Build history of the part. All positions in model axes, mm. A direction names the side the tool comes from. Give positions to 0.01 mm unless a question says otherwise; leave off trailing zeros. Order: outer loops, then holes, each group sorted by start corner. A loop starts at its lowest first (then second) coordinate and runs counter-clockwise, first axis right, second up. Notation, with made-up numbers: (-32, -33.75) -> (-16, -33.75) arc R13 cw to (-16, -29.75) -> close; hole circle Ø10 at (53.25, 40.5). An arc over 180 degrees is marked (long way). One line per item, written item: value. Start each with the question number.
(1) Saw through at A-A on x = 0. Give the cut face in (y, z) (1 decimal).
(2) Two-plate mould, pull along Z, no slides. Class faces 3 (the flat face through (8, 1.905, 208)), 4 (the flat face through (-3, 4.064, -3)): +Z half, -Z half, draft (parallel to the pull), parting line (faces both ways), or undercut.
(3) Pin check, flat tips, straight feed: pin 1 (2.5 mm diameter, centred on x = -23.57, z = 222.46, fed in from +Y); pin 2 (6.5 mm diameter, centred on x = -15, z = 167.17, fed in from -Y). Stop position of each tip, or through.
(4) Which spindle directions (+Z, -Z, +X, -X, +Y, -Y) get a long thin tool onto all of the face, cutting with end or side? Do faces 1 (the cylindrical face through (-193.461, 2.969, -209.304)), 2 (the cylindrical face through (184.75, 0.94, -185.92)). Say none if no direction does.
(5) Probe line 1 (X direction, y = 2.55, z = -199); line 2 (X direction, y = 2.25, z = -104); line 3 (Z direction, x = 24.5, y = 1.4). List the from-to ranges inside material, lowest first.
```python
from build123d import *

# Parameters (mm, degrees)
SKETCH1_W                                           = 457.2
SKETCH1_H                                           = 457.2
BOSS_EXTRUDE1_DEPTH                                 = 4.064
SKETCH2_R                                           = 19.177
CUT_EXTRUDE1_DEPTH                                  = 1.905
CUT_EXTRUDE2_REACH                                  = 4.159
SKETCH3_R                                           = 11.7475
F_10_32_TAPPED_HOLE1_D                              = 4.0386
F_10_32_TAPPED_HOLE2_D                              = 4.0386
CBORE_FOR_10_BINDING_HEAD_MACHINE_SCREW_D           = 5.1054
CBORE_FOR_10_BINDING_HEAD_MACHINE_SCREW_CBORE_D     = 11.1125
CBORE_FOR_10_BINDING_HEAD_MACHINE_SCREW_CBORE_DEPTH = 3.1242
F_1_4_0_25_DIAMETER_HOLE1_D                         = 6.35


with BuildPart() as part:
    # Sketch1 → Boss-Extrude1 (new body)
    with BuildSketch(Plane(origin=(0, 0, 0), x_dir=(1, 0, 0), z_dir=(0, 1, 0))):
        Rectangle(SKETCH1_W, SKETCH1_H)
    extrude(amount=BOSS_EXTRUDE1_DEPTH)

    # Sketch2 → Cut-Extrude1 (cut)
    with BuildSketch(Plane.XZ):
        with Locations((0, 198.882)):
            Circle(SKETCH2_R)
        with Locations((-198.882, -198.882)):
            Circle(SKETCH2_R)
        with Locations((198.882, -198.882)):
            Circle(SKETCH2_R)
    extrude(amount=-CUT_EXTRUDE1_DEPTH, mode=Mode.SUBTRACT)

    # Sketch3 → Cut-Extrude2 (cut, up to next)
    with BuildSketch(Plane.XZ.offset(-1.905), mode=Mode.PRIVATE) as cut_extrude2_sk1:
        with Locations((0, 198.882)):
            Circle(SKETCH3_R)
    cut_extrude2_tool1 = extrude(cut_extrude2_sk1.sketch, amount=-CUT_EXTRUDE2_REACH, mode=Mode.PRIVATE) & part.part
    add(cut_extrude2_tool1.solids().sort_by_distance((0, 1.905, 198.882))[0], mode=Mode.SUBTRACT)
    # Sketch3 → Cut-Extrude2 (cut, up to next)
    with BuildSketch(Plane.XZ.offset(-1.905), mode=Mode.PRIVATE) as cut_extrude2_sk2:
        with Locations((-198.882, -198.882)):
            Circle(SKETCH3_R)
    cut_extrude2_tool2 = extrude(cut_extrude2_sk2.sketch, amount=-CUT_EXTRUDE2_REACH, mode=Mode.PRIVATE) & part.part
    add(cut_extrude2_tool2.solids().sort_by_distance((-198.882, 1.905, -198.882))[0], mode=Mode.SUBTRACT)
    # Sketch3 → Cut-Extrude2 (cut, up to next)
    with BuildSketch(Plane.XZ.offset(-1.905), mode=Mode.PRIVATE) as cut_extrude2_sk3:
        with Locations((198.882, -198.882)):
            Circle(SKETCH3_R)
    cut_extrude2_tool3 = extrude(cut_extrude2_sk3.sketch, amount=-CUT_EXTRUDE2_REACH, mode=Mode.PRIVATE) & part.part
    add(cut_extrude2_tool3.solids().sort_by_distance((198.882, 1.905, -198.882))[0], mode=Mode.SUBTRACT)

    # #10-32 Tapped Hole1 (through all)
    with Locations(Plane(origin=(0, 0, 0), x_dir=(-0.999999981, 0, 0.000197306), z_dir=(0, -1, 0))):
        with Locations((23.617063566, -222.450516863), (-23.529280152, -222.459819113)):
            Hole(F_10_32_TAPPED_HOLE1_D / 2)

    # #10-32 Tapped Hole2 (through all)
    with Locations(Plane(origin=(0, 0, 0), x_dir=(-0.999999981, 0, 0.000197306), z_dir=(0, -1, 0))):
        with Locations((23.607761316, -175.304173145), (-23.538582402, -175.313475395)):
            Hole(F_10_32_TAPPED_HOLE2_D / 2)

    # CBORE for #10 Binding Head Machine Screw1 (through all)
    with Locations(Plane.XZ):
        with Locations((-15, 167.174500066), (15, 167.174500066)):
            CounterBoreHole(CBORE_FOR_10_BINDING_HEAD_MACHINE_SCREW_D / 2, CBORE_FOR_10_BINDING_HEAD_MACHINE_SCREW_CBORE_D / 2, CBORE_FOR_10_BINDING_HEAD_MACHINE_SCREW_CBORE_DEPTH)

    # 1/4 (0.25) Diameter Hole1 (through all)
    with Locations(Plane(origin=(0, 0, 0), x_dir=(-1, 0, 0), z_dir=(0, -1, 0))):
        with Locations((-39.495539735, -58.823311233), (-52.856134437, -37.22112363), (-126.339405298, 81.590908183), (-139.7, 103.193095785), (-139.7, 166.478718596), (-114.3, 166.478718596), (114.3, 166.478718596), (139.7, 166.478718596), (139.7, 103.193095785), (126.339405298, 81.590908183), (52.856134437, -37.22112363), (39.495539735, -58.823311233)):
            Hole(F_1_4_0_25_DIAMETER_HOLE1_D / 2)


solid = part.part
```
Results below:
1. outline: (0, -228.6) -> (4.1, -228.6) -> (4.1, 187.1) -> (1.9, 187.1) -> (1.9, 179.7) -> (0, 179.7) -> close; (0, 218.1) -> (1.9, 218.1) -> (1.9, 210.6) -> (4.1, 210.6) -> (4.1, 228.6) -> (0, 228.6) -> close
2. face 3: undercut
2. face 4: draft
3. pin 1: passes through
3. pin 2: stops at y = 3.12
4. face 1: +Y, -Y
4. face 2: -Y
5. line 1: x = -228.6 to -210.63, -187.14 to 187.14, 210.63 to 228.6
5. line 2: x = -228.6 to -142.77, -136.63 to 136.63, 142.77 to 228.6
5. line 3: z = -228.6 to 173.51, 177.1 to 220.66, 224.25 to 228.6
